Part model, mm, in its own coordinate system. A direction names the side the tool comes from. Give positions to 0.01 mm unless a question says otherwise; leave off trailing zeros. Loops run counter-clockwise (first coordinate to the right, second up) from the corner with the lowest first, then second, coordinate; pieces in that order, holes last. Notation, with made-up numbers: (-11.5, 87.5) -> (17.5, 87.5) arc R28 ccw to (17.5, 107.5) -> close; hole circle Ø2 at (-25, 25). An arc over 180 degrees is marked (long way). Write item = value, one per line.
from build123d import *

# Parameters (mm, degrees)
F1_DEPTH = 508
F3_D     = 26.9875
F3_DEPTH = 25.4


with BuildPart() as f1:
    # F0 (on Front) → F1 (new body, symmetric)
    with BuildSketch(Plane.XZ):
        with BuildLine():
            Line((127, -228.6), (127, -203.2))
            Line((127, -203.2), (12.065, -203.2))
            ThreePointArc((12.065, -203.2), (10.268949, -202.456051), (9.525, -200.66))
            Line((9.525, -200.66), (9.525, 200.66))
            ThreePointArc((9.525, 200.66), (10.268949, 202.456051), (12.065, 203.2))
            Line((12.065, 203.2), (127, 203.2))
            Line((127, 203.2), (127, 228.6))
            Line((127, 228.6), (-127, 228.6))
            Line((-127, 228.6), (-127, 203.2))
            Line((-127, 203.2), (-12.065, 203.2))
            ThreePointArc((-12.065, 203.2), (-10.268949, 202.456051), (-9.525, 200.66))
            Line((-9.525, 200.66), (-9.525, -200.66))
            ThreePointArc((-9.525, -200.66), (-10.268949, -202.456051), (-12.065, -203.2))
            Line((-12.065, -203.2), (-127, -203.2))
            Line((-127, -203.2), (-127, -228.6))
            Line((-127, -228.6), (127, -228.6))
        make_face()
    extrude(amount=F1_DEPTH, both=True)

    # F3
    with Locations(Plane.XY.offset(228.6)):
        with Locations((-66.675, 141.293497), (-66.675, 65.093497), (-66.675, -11.106503), (-66.675, -87.306503), (66.675, -87.306503), (66.675, -11.106503), (66.675, 65.093497), (66.675, 141.293497)):
            Hole(F3_D / 2, depth=F3_DEPTH)


solid = f1.part
1) Drill centre lines: line 1 along Z through (x, y) = (-34, -403); line 2 along X through (y, z) = (-338, 182.5) (3 decimals). Where is each one in solid material? Low to high. Write a range as [from, to].
Resolved:
line_1 = [-228.6, -203.2], [203.2, 228.6]
line_2 = [-9.525, 9.525]
2) Slice it at B-B, the plane y = -345. List the corners of the cut face in (x, z) (3 decimals).
Resolved:
outline = (-127, -228.6) -> (127, -228.6) -> (127, -203.2) -> (12.065, -203.2) arc R2.54 cw to (9.525, -200.66) -> (9.525, 200.66) arc R2.54 cw to (12.065, 203.2) -> (127, 203.2) -> (127, 228.6) -> (-127, 228.6) -> (-127, 203.2) -> (-12.065, 203.2) arc R2.54 cw to (-9.525, 200.66) -> (-9.525, -200.66) arc R2.54 cw to (-12.065, -203.2) -> (-127, -203.2) -> close
3) Slice it at C-C, the plane z = -74. List the corners of the cut face in (x, y) (3 decimals), and give its area (3 significant figures).
Resolved:
outline = (-9.525, -508) -> (9.525, -508) -> (9.525, 508) -> (-9.525, 508) -> close
area = 19,400 mm²
4) Which spindle directions (+Z, -Z, +X, -X, +Y, -Y) get a long thin tool onto all of the face, cutting with end or side? Do faces 5 (the face through (-83, -7, 203.2)), 6 (the face through (-127, -7, 216)), 7 (the face through (76.62, 74.213, 215.722)), 8 (the face through (9.525, -7, -3)). Say none if no direction does.
Resolved:
face_5 = -X, +Y, -Y
face_6 = +Z, -Z, -X, +Y, -Y
face_7 = +Z
face_8 = +X, +Y, -Y
5) Slice it at A-A, the plane x = 40. List the corners of the cut face in (y, z), and give its area (3 significant figures).
Resolved:
outline = (-508, -228.6) -> (508, -228.6) -> (508, -203.2) -> (-508, -203.2) -> close; (-508, 203.2) -> (508, 203.2) -> (508, 228.6) -> (-508, 228.6) -> close
area = 51,600 mm²
6) Drop flat-ended pins along their axis: P1, Ø24.5, axis at x = 66.68, y = 141.29, coming from the +Z side; P2, Ø4, axis at y = -180.5, z = 116, coming from the +X side (3 decimals); P3, Ø1.5, axis at y = -341.5, z = 104.5, coming from the -X side (3 decimals); P4, Ø8, axis at x = -14.5, z = 104.5, coming from the -Y side. Give the stop position or say it passes through.
Resolved:
P1 = -203.2
P2 = 9.525
P3 = -9.525
P4 = through
7) Pull direction Z, two halves, no side cores. Call faces 1 (the face through (-2, -7, -228.6)), 2 (the face through (81, -7, 203.2)), 3 (the face through (2, -7, 228.6)), 4 (the face through (76.62, -78.187, 215.722)): pulls with the +Z half, pulls with the -Z half, needs draft (parallel to the pull), parting line crosses it, or undercut.
Resolved:
face_1 = pulls with the -Z half
face_2 = undercut
face_3 = pulls with the +Z half
face_4 = needs draft
